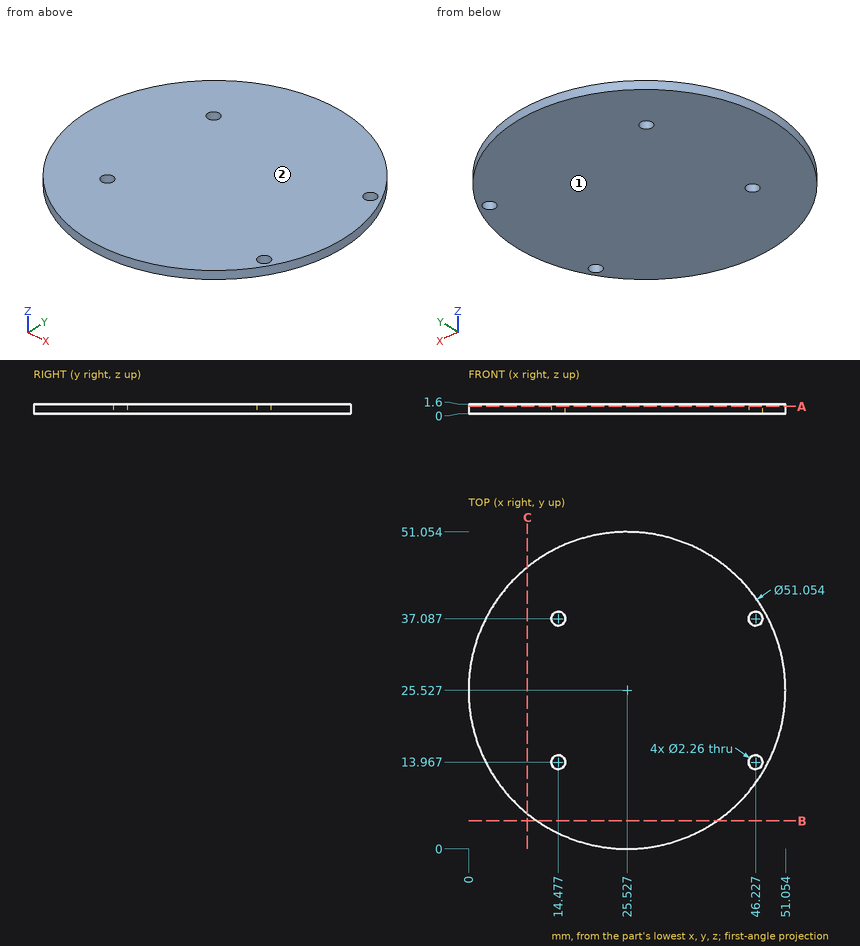
Verification items for this drawing (mm, ordinates from the low corner). Give positions to 0.01 mm unless a question says otherwise; leave off trailing zeros. Write each loop counter-clockwise with the first axis right and the second up, starting at its lowest first coordinate (ties: lowest second). Pieces come first, ordered by that corner, then holes. Notation, with made-up numbers: (20, 39.25) -> (57, 39.25) arc R15 ccw to (57, 51.25) -> close; hole circle Ø2 at (53, 54.25). An arc over 180 degrees is marked (long way). Use one line per item in the form item = value.
Item 1: Sectioned sample at B-B on y = 4.5. Enter the section's corners in (x, z).
Results list:
outline = (11.05, 0) -> (40, 0) -> (40, 1.6) -> (11.05, 1.6) -> close
Item 2: Sectioned sample at C-C on x = 9.5. Enter the section's corners in (y, z).
Results list:
outline = (5.66, 0) -> (45.4, 0) -> (45.4, 1.6) -> (5.66, 1.6) -> close
Item 3: Scan lines: line 1 (X direction, y = 14.5, z = 0.8); line 2 (X direction, y = 38, z = 1.1); line 3 (Y direction, x = 26, z = 1.05). Record each from-to range of solid material in increasing order.
Results list:
line_1 = 2.5 to 13.48, 15.47 to 45.23, 47.22 to 48.55
line_2 = 3.25 to 13.81, 15.14 to 45.56, 46.89 to 47.8
line_3 = 0 to 51.05
Item 4: Depth check by flat-ended pin: pin 1 Ø1.8 at (x, y) = (14.477, 13.967) entering from +Z. Enter the tip coordinate at first touch or a pass-through.
Results list:
pin_1 = through
Item 5: Mould release check, pull along Z, two halves, no side actions. Record for the marked faces 1 and 2: released by +Z, released by -Z, zero draft, split by the parting line, or undercut.
Results list:
face_1 = released by -Z
face_2 = released by +Z
Item 6: Sectioned sample at A-A on z = 1.2. Enter the section's corners in (x, y), plus the area to 3 significant figures.
Results list:
outline = circle Ø51.05 at (25.53, 25.53); hole circle Ø2.26 at (14.48, 13.97); hole circle Ø2.26 at (14.48, 37.09); hole circle Ø2.26 at (46.23, 13.97); hole circle Ø2.26 at (46.23, 37.09)
area = 2,030 mm2
